CAD build for the part. Positions are in the model's coordinates, mm. A direction names the side the tool comes from. Coordinates: 2 decimals unless noted, no trailing zeros. Loops run counter-clockwise (first coordinate to the right, second up) from the corner with the lowest first, then second, coordinate; pieces in that order, holes last. Notation, with made-up numbers: (84.25, 23.5) -> (138.25, 23.5) arc R19 ccw to (138.25, 52.5) -> close; hole circle Ø8 at (32.25, 42). An arc over 180 degrees is marked (long way). Write each question's results on one line, items separated by ' | '.
```python
from build123d import *

# Parameters (mm, degrees)
SKETCH1_W           = 49.87
SKETCH1_H           = 146.11
BOSS_EXTRUDE1_DEPTH = 41.6
SKETCH2_W           = 49.87
SKETCH2_H           = 41.6
BOSS_EXTRUDE2_DEPTH = 21.57
FILLET2_R           = 15
SKETCH6_R           = 2.305
BOSS_EXTRUDE4_DEPTH = 8
SKETCH7_R           = 2.305
BOSS_EXTRUDE5_DEPTH = 8
SKETCH8_W           = 1.72
SKETCH8_H           = 7.3
BOSS_EXTRUDE6_DEPTH = 8
FILLET3_R           = 2


with BuildPart() as part:
    # Sketch1 → Boss-Extrude1 (new body)
    with BuildSketch(Plane(origin=(0, 0, 0), x_dir=(1, 0, 0), z_dir=(0, 1, 0))):
        Rectangle(SKETCH1_W, SKETCH1_H)
    extrude(amount=BOSS_EXTRUDE1_DEPTH)

    # Sketch2 → Boss-Extrude2 (add)
    with BuildSketch(Plane.XY.offset(73.055)):
        with Locations((0.021729079, 20.81046652)):
            Rectangle(SKETCH2_W, SKETCH2_H)
    extrude(amount=BOSS_EXTRUDE2_DEPTH)

    # Fillet2
    fillet2_edges = [part.edges().sort_by_distance(p)[0] for p in [
        (0.021729079, 0.01046652, 94.625),
        (0.021729079, 41.61046652, 94.625),
    ]]
    fillet(fillet2_edges, radius=FILLET2_R)

    # Sketch6 → Boss-Extrude4 (add)
    with BuildSketch(Plane.XY.offset(94.625)):
        with Locations((-22.382137535, 24.07655878)):
            Circle(SKETCH6_R)
    extrude(amount=BOSS_EXTRUDE4_DEPTH)

    # Sketch7 → Boss-Extrude5 (add)
    with BuildSketch(Plane.XY.offset(94.625)):
        with Locations((-22.226360129, 18.312794768)):
            Circle(SKETCH7_R)
    extrude(amount=BOSS_EXTRUDE5_DEPTH)

    # Sketch8 → Boss-Extrude6 (add)
    with BuildSketch(Plane.XY.offset(94.625)):
        with Locations((22.28703356, 20.493678449)):
            Rectangle(SKETCH8_W, SKETCH8_H)
    extrude(amount=BOSS_EXTRUDE6_DEPTH)

    # Fillet3
    fillet3_edges = [part.edges().sort_by_distance(p)[0] for p in [
        (0, 41.6, -73.055),
        (0, 0, -73.055),
    ]]
    fillet(fillet3_edges, radius=FILLET3_R)


solid = part.part
```
Q1. Drop flat-ended pins along their axis: pin 1 (4 mm diameter, centred on y = 20, z = 51, fed in from +X) (3 decimals); pin 2 (1.4 mm diameter, centred on x = 22.5, z = 100, fed in from -Y); pin 3 (2 mm diameter, centred on x = -2, z = -14.5, fed in from +Y). Give the stop position or say it passes through.
Results are:
pin 1: x = 24.935 | pin 2: y = 16.84 | pin 3: y = 41.6
Q2. Cut at A-A on x = 16. Write the cut outline in (y, z) (3 decimals), and give its area (3 significant figures).
Results are:
outline: (0, -71.055) arc R2 ccw to (2, -73.055) -> (39.6, -73.055) arc R2 ccw to (41.6, -71.055) -> (41.6, 73.055) -> (41.61, 73.055) -> (41.61, 79.625) arc R15 ccw to (26.61, 94.625) -> (15.01, 94.625) arc R15 ccw to (0.01, 79.625) -> (0.01, 73.055) -> (0, 73.055) -> close | area: 6,880 mm^2
Q3. Which spindle directions (+Z, -Z, +X, -X, +Y, -Y) get a long thin tool onto all of the face, cutting with end or side? Do faces 5 (the flat face through (21.427, 20, 99)), 6 (the flat face through (0, 0.01, 76)), 7 (the flat face through (23.147, 20, 99)). Say none if no direction does.
Results are:
face 5: +Z, +Y, -Y | face 6: +Z, -Z, +X, -X, -Y | face 7: +Z, +X, +Y, -Y
Q4. Cut at B-B on y = 7. Write the cut outline in (x, z) (3 decimals), and give its area (3 significant figures).
Results are:
outline: (-24.935, -73.055) -> (24.935, -73.055) -> (24.935, 73.055) -> (24.957, 73.055) -> (24.957, 92.307) -> (-24.913, 92.307) -> (-24.913, 73.055) -> (-24.935, 73.055) -> close | area: 8,250 mm^2
Q5. Pull direction Y, two halves, no side cores. Call faces 1 (the cylindrical face through (0.371, 4.288, 90.114)), 2 (the flat face through (0, 41.61, 76)), 3 (the cylindrical face through (-20.097, 17.43, 98.569)), 4 (the cylindrical face through (-24.081, 25.634, 98.569)): +Y half, -Y half, draft (parallel to the pull), parting line (faces both ways), or undercut.
Results are:
face 1: -Y half | face 2: +Y half | face 3: undercut | face 4: undercut
Q6. Cut at C-C on y = 36. Write the cut outline in (x, z) (3 decimals), and give its area (3 significant figures).
Results are:
outline: (-24.935, -73.055) -> (24.935, -73.055) -> (24.935, 73.055) -> (24.957, 73.055) -> (24.957, 91.323) -> (-24.913, 91.323) -> (-24.913, 73.055) -> (-24.935, 73.055) -> close | area: 8,200 mm^2
Q7. Wall check: L1, parallel to Y at x = -8, z = -30.5; L2, parallel to Z at x = 14, y = 14.5 (3 decimals); L3, parallel to X at y = 25, z = 79. Give the ranges that are in metal, low to high. Write a range as from..to.
Results are:
L1: 0..41.6 | L2: -73.055..94.616 | L3: -24.91..24.96
